Read the model definition and answer for the solid it produces. Units are mm, in the model's axes. Face numbers are marked on the shaded views. A direction names the side the tool comes from. Round coordinates to 2 decimals unless told otherwise and drop trailing zeros. Loops run counter-clockwise (first coordinate to the right, second up) from the corner with the lowest first, then second, coordinate; pieces in that order, holes last. Notation, with made-up numbers: (-24, 63.25) - (-6, 63.25) arc R26 cw to (-6, 96.25) - close; hole circle Ø11 at (80, -28.5). An arc over 180 degrees is marked (long way). Answer as CSV lines item,"result".
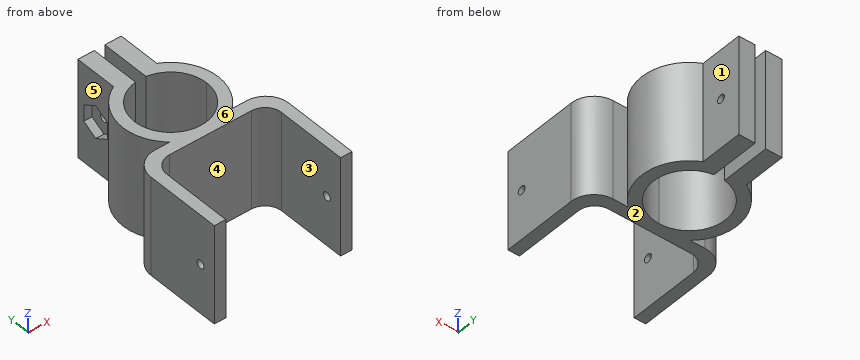
```python
from build123d import *

# Parameters (mm, degrees)
F1_DEPTH = 38.1
F2_R     = 1.5875
F3_DEPTH = 35.053
F4_R     = 1.5875
F5_DEPTH = 3.175
F6_R     = 1.5875
F7_DEPTH = 53.341


with BuildPart() as f1:
    # F0 (on Top) → F1 (new body)
    with BuildSketch(Plane.XY):
        with BuildLine():
            Line((-11.9979717036, 0), (-17.78, 0))
            ThreePointArc((-17.78, 0), (-24.0661792847, -2.6038207153), (-26.67, -8.89))
            Line((-26.67, -8.89), (-26.67, -38.1))
            Line((-26.67, -38.1), (-22.225, -38.1))
            Line((-22.225, -38.1), (-22.225, -10.795))
            ThreePointArc((-22.225, -10.795), (-20.3651280605, -6.3048719395), (-15.875, -4.445))
            Line((-15.875, -4.445), (-2.57e-08, -4.445))
            ThreePointArc((-2.57e-08, -4.445), (-6.3974477453, -3.2980307895), (-11.9979717036, 0))
        make_face()
        with BuildLine():
            Line((9.2e-09, 0), (-11.9979717036, 0))
            ThreePointArc((-11.9979717036, 0), (-6.3974477453, -3.2980307895), (-2.57e-08, -4.445))
            ThreePointArc((-2.57e-08, -4.445), (6.3974477212, -3.2980307984), (11.9979717036, 0))
            Line((11.9979717036, 0), (9.2e-09, 0))
        make_face()
        with BuildLine():
            ThreePointArc((11.9979717036, 0), (6.3974477212, -3.2980307984), (-2.57e-08, -4.445))
            Line((-2.57e-08, -4.445), (15.875, -4.445))
            ThreePointArc((15.875, -4.445), (20.3651280605, -6.3048719395), (22.225, -10.795))
            Line((22.225, -10.795), (22.225, -38.1))
            Line((22.225, -38.1), (26.67, -38.1))
            Line((26.67, -38.1), (26.67, -8.89))
            ThreePointArc((26.67, -8.89), (24.0661792847, -2.6038207153), (17.78, 0))
            Line((17.78, 0), (11.9979717036, 0))
        make_face()
        with BuildLine():
            ThreePointArc((13.97, 13.97), (9.8782817364, 4.0917182701), (9.2e-09, 0))
            Line((9.2e-09, 0), (11.9979717036, 0))
            ThreePointArc((11.9979717036, 0), (16.7340203466, 6.2833370024), (18.415, 13.97))
            ThreePointArc((18.415, 13.97), (15.7077489635, 23.5813915486), (8.382, 30.3667771528))
            Line((8.382, 30.3667771528), (8.382, 27.7914281462))
            Line((8.382, 27.7914281462), (2.032, 27.7914281462))
            ThreePointArc((2.032, 27.7914281462), (10.5723209372, 23.1016444302), (13.97, 13.97))
        make_face()
        with BuildLine():
            ThreePointArc((-8.382, 30.3667771528), (-18.285816917, 16.1474123812), (-11.9979717036, 0))
            Line((-11.9979717036, 0), (9.2e-09, 0))
            ThreePointArc((9.2e-09, 0), (-13.9328075273, 12.9512878678), (-2.032, 27.7914281462))
            Line((-2.032, 27.7914281462), (-8.382, 27.7914281462))
            Line((-8.382, 27.7914281462), (-8.382, 30.3667771528))
        make_face()
        with BuildLine():
            Line((2.032, 32.2725462983), (2.032, 27.7914281462))
            Line((2.032, 27.7914281462), (8.382, 27.7914281462))
            Line((8.382, 27.7914281462), (8.382, 30.3667771528))
            ThreePointArc((8.382, 30.3667771528), (5.2934712627, 31.6077829387), (2.032, 32.2725462983))
        make_face()
        with BuildLine():
            Line((2.032, 46.8414281462), (2.032, 32.2725462983))
            ThreePointArc((2.032, 32.2725462983), (5.2934712627, 31.6077829387), (8.382, 30.3667771528))
            Line((8.382, 30.3667771528), (8.382, 46.8414281462))
            Line((8.382, 46.8414281462), (2.032, 46.8414281462))
        make_face()
        with BuildLine():
            ThreePointArc((-2.032, 32.2725462983), (-5.2934712627, 31.6077829387), (-8.382, 30.3667771528))
            Line((-8.382, 30.3667771528), (-8.382, 27.7914281462))
            Line((-8.382, 27.7914281462), (-2.032, 27.7914281462))
            Line((-2.032, 27.7914281462), (-2.032, 32.2725462983))
        make_face()
        with BuildLine():
            Line((-8.382, 46.8414281462), (-8.382, 30.3667771528))
            ThreePointArc((-8.382, 30.3667771528), (-5.2934712627, 31.6077829387), (-2.032, 32.2725462983))
            Line((-2.032, 32.2725462983), (-2.032, 46.8414281462))
            Line((-2.032, 46.8414281462), (-8.382, 46.8414281462))
        make_face()
    extrude(amount=F1_DEPTH)

    # F2 (on face) → F3 (cut, through all)
    with BuildSketch(Plane.YZ.offset(8.382)):
        with Locations((38.6041026495, 19.05)):
            Circle(F2_R)
    extrude(amount=-F3_DEPTH, mode=Mode.SUBTRACT)

    # F4 (on face) → F5 (cut)
    with BuildSketch(Plane(origin=(-8.382, 0, 0), x_dir=(0, -1, 0), z_dir=(-1, 0, 0))):
        Polygon((-44.1033639635, 22.225), (-44.1033639635, 15.875), (-38.6041026495, 12.7), (-33.1048413355, 15.875), (-33.1048413355, 22.225), (-38.6041026495, 25.4), align=None)
        with Locations((-38.6041026495, 19.05)):
            Circle(F4_R, mode=Mode.SUBTRACT)
    extrude(amount=-F5_DEPTH, mode=Mode.SUBTRACT)

    # F6 (on face) → F7 (cut, through all)
    with BuildSketch(Plane(origin=(-26.67, 0, 0), x_dir=(0, -1, 0), z_dir=(-1, 0, 0))):
        with Locations((31.75, 19.05)):
            Circle(F6_R)
    extrude(amount=-F7_DEPTH, mode=Mode.SUBTRACT)


solid = f1.part
```
1) A tool of negligible diameter and unlimited length cuts with its end or side. For the marked faces 4, 5 and 6, from which of +Z, -Z, +X, -X, +Y, -Y can it reach the whole face along a straight path? Write none if from no direction.
Entries:
face 4,"+Z, -Z, -Y"
face 5,"+Z, -Z, -X, +Y"
face 6,"+Z, +X, -X, +Y, -Y"
2) A cutting plane is placed at D-D, the plane z = 9. Determine the outline of the cut face in (x, y) (3 decimals).
Entries:
outline,"(-26.67, -38.1) - (-22.225, -38.1) - (-22.225, -10.795) arc R6.35 cw to (-15.875, -4.445) - (15.875, -4.445) arc R6.35 cw to (22.225, -10.795) - (22.225, -38.1) - (26.67, -38.1) - (26.67, -8.89) arc R8.89 ccw to (17.78, 0) - (11.998, 0) arc R18.415 ccw to (8.382, 30.367) - (8.382, 46.841) - (2.032, 46.841) - (2.032, 27.791) arc R13.97 cw (long way) to (-2.032, 27.791) - (-2.032, 46.841) - (-8.382, 46.841) - (-8.382, 30.367) arc R18.415 ccw to (-11.998, 0) - (-17.78, 0) arc R8.89 ccw to (-26.67, -8.89) - close"
3) Find the intervals of material crossed by line 1 (Z direction, x = 23.4, y = -31.75); line 2 (X direction, y = 13.5, z = 21.5); line 3 (X direction, y = -24, z = 21.5) (3 decimals), in increasing order.
Entries:
line 1,"z = 0 to 17.46, 20.64 to 38.1"
line 2,"x = -18.41 to -13.96, 13.96 to 18.41"
line 3,"x = -26.67 to -22.225, 22.225 to 26.67"
4) The mould has two halves that part along X. Classify the marked faces 1, 2 and 3: pulls with the +X half, pulls with the -X half, needs draft (parallel to the pull), parting line crosses it, or undercut.
Entries:
face 1,"pulls with the +X half"
face 2,"needs draft"
face 3,"undercut"
5) Each of these flat-tipped pins is pushed along its axis until it touches: P1, Ø3, axis at x = 11.5, z = 32.5, coming from the -Y side (3 decimals); P2, Ø12, axis at x = -18.5, y = 35, coming from the -Z side; P3, Ø6.5, axis at x = -16.5, z = 22, coming from the +Y side; P4, Ø3.5, axis at y = 36.5, z = 17, coming from the -X side. Where does it stop, or does it pass through?
Entries:
P1,"stops at y = -4.445"
P2,"passes through"
P3,"stops at y = 26.76"
P4,"stops at x = -5.21"
6) A cutting plane is placed at B-B, the plane y = -31.75. Determine the outline of the cut face in (x, z) (1 decimal), plus the area to 3 significant figures.
Entries:
outline,"(-26.7, 0) - (-22.2, 0) - (-22.2, 17.5) - (-26.7, 17.5) - close; (-26.7, 20.6) - (-22.2, 20.6) - (-22.2, 38.1) - (-26.7, 38.1) - close; (22.2, 0) - (26.7, 0) - (26.7, 17.5) - (22.2, 17.5) - close; (22.2, 20.6) - (26.7, 20.6) - (26.7, 38.1) - (22.2, 38.1) - close"
area,"310 mm^2"
7) A cutting plane is placed at C-C, the plane x = 6. Count the separate pieces of the cut face and the enclosed holes in it, plus the area to 3 significant figures.
Entries:
separate pieces,"2"
enclosed holes,"1"
area,"985 mm^2"
8) A cutting plane is placed at A-A, the plane y = -13.5. Determine the outline of the cut face in (x, z) (3 decimals).
Entries:
outline,"(-26.67, 0) - (-22.225, 0) - (-22.225, 38.1) - (-26.67, 38.1) - close; (22.225, 0) - (26.67, 0) - (26.67, 38.1) - (22.225, 38.1) - close"
